Work out the finished part from the listing and answer in its coordinate system (mm). A direction names the side the tool comes from. Give positions to 0.01 mm unless a question says otherwise; leave off trailing zeros. Order: outer loops, then holes, each group sorted by start corner. A loop starts at its lowest first (then second) coordinate and runs counter-clockwise, first axis right, second up. Notation, with made-up numbers: (-7.5, 18.5) - (0.5, 18.5) arc R26 ccw to (0.5, 52.5) - close; hole circle Ø6 at (-20, -32). An arc over 180 degrees is marked (long way). Put each result on its own line as item: value.
```python
from build123d import *

# Parameters (mm, degrees)
F0_R     = 1.63195
F1_DEPTH = 1.5
F2_W     = 6.985
F2_H     = 6.985
F2_R     = 0.746035
F2_W_2   = 7.13823
F2_W_3   = 5.5
F2_H_2   = 5.5
F3_DEPTH = 9
F4_DEPTH = 3.7


with BuildPart() as f1:
    # F0 (on Top) → F1 (new body)
    with BuildSketch(Plane.XY):
        with BuildLine():
            Line((0.45623, 22.43354), (-28.65877, 22.43354))
            ThreePointArc((-28.65877, 22.43354), (-29.365876, 22.140646), (-29.65877, 21.43354))
            Line((-29.65877, 21.43354), (-29.65877, 18.35354))
            ThreePointArc((-29.65877, 18.35354), (-29.365876, 17.646433), (-28.65877, 17.35354))
            Line((-28.65877, 17.35354), (-24.57877, 17.35354))
            Line((-24.57877, 17.35354), (-24.57877, -6.41146))
            ThreePointArc((-24.57877, -6.41146), (-24.285876, -7.118567), (-23.57877, -7.41146))
            Line((-23.57877, -7.41146), (5.53623, -7.41146))
            ThreePointArc((5.53623, -7.41146), (6.243337, -7.118567), (6.53623, -6.41146))
            Line((6.53623, -6.41146), (6.53623, -3.33146))
            ThreePointArc((6.53623, -3.33146), (6.243337, -2.624354), (5.53623, -2.33146))
            Line((5.53623, -2.33146), (1.45623, -2.33146))
            Line((1.45623, -2.33146), (1.45623, 21.43354))
            ThreePointArc((1.45623, 21.43354), (1.163337, 22.140646), (0.45623, 22.43354))
        make_face()
        with Locations((3.99623, -4.87146)):
            Circle(F0_R, mode=Mode.SUBTRACT)
        with Locations((-27.11877, 19.89354)):
            Circle(F0_R, mode=Mode.SUBTRACT)
    extrude(amount=F1_DEPTH)

    # F2 (on face) → F3 (join)
    with BuildSketch(Plane.XY.offset(1.5)):
        with Locations((-19.94327, 18.94104)):
            Rectangle(F2_W, F2_H)
        with Locations((-21.915814, 18.94104)):
            Circle(F2_R, mode=Mode.SUBTRACT)
        with Locations((-18.583925, 18.94104)):
            Circle(F2_R, mode=Mode.SUBTRACT)
        with Locations((-11.56127, 18.94104)):
            Rectangle(F2_W, F2_H)
        with Locations((-13.293799, 18.94104)):
            Circle(F2_R, mode=Mode.SUBTRACT)
        with Locations((-9.818212, 18.94104)):
            Circle(F2_R, mode=Mode.SUBTRACT)
        with Locations((-3.17927, 18.94104)):
            Rectangle(F2_W, F2_H)
        with Locations((-4.874569, 18.94104)):
            Circle(F2_R, mode=Mode.SUBTRACT)
        with Locations((-1.815664, 18.94104)):
            Circle(F2_R, mode=Mode.SUBTRACT)
        with Locations((-3.255885, -3.91896)):
            Rectangle(F2_W_2, F2_H)
        with Locations((-4.876917, -5.169022)):
            Circle(F2_R, mode=Mode.SUBTRACT)
        with Locations((-1.506733, -5.169022)):
            Circle(F2_R, mode=Mode.SUBTRACT)
        with Locations((-12.551931, -4.66146)):
            Rectangle(F2_W_3, F2_H_2)
        with Locations((-13.975609, -5.169022)):
            Circle(F2_R, mode=Mode.SUBTRACT)
        with Locations((-11.063594, -5.169022)):
            Circle(F2_R, mode=Mode.SUBTRACT)
        with Locations((-19.13806, -4.66146)):
            Rectangle(F2_W_3, F2_H_2)
        with Locations((-20.561739, -5.169022)):
            Circle(F2_R, mode=Mode.SUBTRACT)
        with Locations((-17.649723, -5.169022)):
            Circle(F2_R, mode=Mode.SUBTRACT)
    extrude(amount=F3_DEPTH)

    # F2 (on face) → F4 (join)
    with BuildSketch(Plane.XY.offset(1.5)):
        with Locations((-20.561739, -5.169022)):
            Circle(F2_R)
        with Locations((-13.975609, -5.169022)):
            Circle(F2_R)
        with Locations((-17.649723, -5.169022)):
            Circle(F2_R)
        with Locations((-11.063594, -5.169022)):
            Circle(F2_R)
        with Locations((-4.876917, -5.169022)):
            Circle(F2_R)
        with Locations((-1.506733, -5.169022)):
            Circle(F2_R)
        with Locations((-1.815664, 18.94104)):
            Circle(F2_R)
        with Locations((-4.874569, 18.94104)):
            Circle(F2_R)
        with Locations((-9.818212, 18.94104)):
            Circle(F2_R)
        with Locations((-18.583925, 18.94104)):
            Circle(F2_R)
        with Locations((-21.915814, 18.94104)):
            Circle(F2_R)
    extrude(amount=-F4_DEPTH)


solid = f1.part
```
(1) Straight lines are drawn through the part: line 1 (Y direction, x = -4, z = 7.5); line 2 (Y direction, x = -13, z = 2); line 3 (Z direction, x = -17, y = 7). For each, find the intervals that lie inside material, in ascending order.
Geometry check:
line 1: y = -7.41 to -0.43, 15.45 to 22.43
line 2: y = -7.41 to -1.91, 15.45 to 18.26, 19.63 to 22.43
line 3: z = 0 to 1.5
(2) Given pin 1 (2 mm diameter, centred on y = 19.5, z = 5.5, fed in from +X); pin 2 (5.5 mm diameter, centred on y = 20, z = 7, fed in from -X); pin 3 (4 mm diameter, centred on y = 4, z = 2, fed in from +X), each flat-ended and moving along its own axis, determine where each tip first touches the part or whether it passes through.
Geometry check:
pin 1: stops at x = 0.31
pin 2: stops at x = -23.44
pin 3: stops at x = 1.46
(3) Section A-A, the plane x = -3.5 is taken. Write down the section's boundary in (y, z), then the cut area to 3 significant figures.
Geometry check:
outline: (-7.41, 0) - (22.43, 0) - (22.43, 10.5) - (15.45, 10.5) - (15.45, 1.5) - (-0.43, 1.5) - (-0.43, 10.5) - (-7.41, 10.5) - close
area: 170 mm²
(4) Section C-C, the plane y = 20.75 is taken. Write down the section's boundary in (x, z).
Geometry check:
outline: (-29.66, 0) - (-28.51, 0) - (-28.51, 1.5) - (-29.66, 1.5) - close; (-25.73, 0) - (1.46, 0) - (1.46, 1.5) - (0.31, 1.5) - (0.31, 10.5) - (-6.67, 10.5) - (-6.67, 1.5) - (-8.07, 1.5) - (-8.07, 10.5) - (-15.05, 10.5) - (-15.05, 1.5) - (-16.45, 1.5) - (-16.45, 10.5) - (-23.44, 10.5) - (-23.44, 1.5) - (-25.73, 1.5) - close
(5) Section D-D, the plane y = 16.5 is taken. Write down the section's boundary in (x, z).
Geometry check:
outline: (-24.58, 0) - (1.46, 0) - (1.46, 1.5) - (0.31, 1.5) - (0.31, 10.5) - (-6.67, 10.5) - (-6.67, 1.5) - (-8.07, 1.5) - (-8.07, 10.5) - (-15.05, 10.5) - (-15.05, 1.5) - (-16.45, 1.5) - (-16.45, 10.5) - (-23.44, 10.5) - (-23.44, 1.5) - (-24.58, 1.5) - close
(6) Determine the mould class of faces 1 (the face through (-16.451, 19, 6)), 2 (the face through (-3, -0.426, 6)), 3 (the face through (6.536, -5, 1)), 4 (the face through (-6.825, -4, 6)) for opening direction X: pulls with the +X half, pulls with the -X half, needs draft (parallel to the pull), parting line crosses it, or undercut.
Geometry check:
face 1: undercut
face 2: needs draft
face 3: pulls with the +X half
face 4: undercut
(7) Section B-B, the plane z = -1 is taken. Count the separate pieces of the cut face and the enclosed holes in it, then the cut area to 3 significant figures.
Geometry check:
separate pieces: 11
enclosed holes: 0
area: 19.2 mm²
(8) A tool of negligible diameter and unlimited length cuts with its end or side. For faces 5 (the face through (-18.2, 18.3, -1.1)), 6 (the face through (-18.395, -5.136, 5.937)), 7 (the face through (-15.302, -5, 6)), 8 (the face through (-9.802, -5, 6)), from which of +Z, -Z, +X, -X, +Y, -Y can it reach the whole face along a straight path? Write none if from no direction.
Geometry check:
face 5: -Z
face 6: +Z
face 7: +Z, +Y, -Y
face 8: +Z, -Y
